Part model, mm, in its own coordinate system. A direction names the side the tool comes from. Round coordinates to 2 decimals unless told otherwise and drop trailing zeros. Write each loop counter-clockwise with the first axis right and the second up, starting at its lowest first coordinate (ties: lowest second). Pieces come first, ordered by that corner, then holes. Notation, with made-up numbers: (45, 31) -> (71, 31) arc R15 cw to (71, 41) -> close; hole circle Ø7 at (-3.5, -32). An arc over 180 degrees is marked (long way). Return JSON: item names as keys, results as strings. Group by question number.
```python
from build123d import *

# Parameters (mm, degrees)
SKETCH1_W                = 25
SKETCH1_H                = 25
BOSS_EXTRUDE1_DEPTH      = 30
SKETCH6_W                = 15
SKETCH6_H                = 15
BOSS_EXTRUDE2_DEPTH      = 8
BOSS_EXTRUDE2_DEPTH_BACK = 12
SKETCH3_R                = 2.5
CUT_EXTRUDE1_DEPTH       = 13.5
CUT_EXTRUDE1_DEPTH_BACK  = 13.5
SKETCH5_R                = 6
CUT_EXTRUDE4_DEPTH       = 11
SKETCH2_R                = 3
CUT_EXTRUDE6_DEPTH       = 31
SKETCH4_R                = 4.25
CUT_EXTRUDE3_DEPTH       = 17.5
FILLET1_R                = 5
FILLET2_R                = 2


with BuildPart() as part:
    # Sketch1 → Boss-Extrude1 (new body)
    with BuildSketch(Plane(origin=(0, 0, 0), x_dir=(1, 0, 0), z_dir=(0, 1, 0))):
        Rectangle(SKETCH1_W, SKETCH1_H)
    extrude(amount=-BOSS_EXTRUDE1_DEPTH)

    # Sketch6 → Boss-Extrude2 (add, two sides)
    with BuildSketch(Plane(origin=(0, 0, 0), x_dir=(1, 0, 0), z_dir=(0, 1, 0))) as boss_extrude2_sk:
        with Locations((20, 5)):
            Rectangle(SKETCH6_W, SKETCH6_H)
        with Locations((-20, 5)):
            Rectangle(SKETCH6_W, SKETCH6_H)
    extrude(amount=BOSS_EXTRUDE2_DEPTH)
    extrude(boss_extrude2_sk.sketch, amount=-BOSS_EXTRUDE2_DEPTH_BACK)

    # Sketch3 → Cut-Extrude1 (cut, two sides)
    with BuildSketch(Plane.XY) as cut_extrude1_sk:
        with Locations((0, -20)):
            Circle(SKETCH3_R)
        with Locations((20, 0)):
            Circle(SKETCH3_R)
        with Locations((-20, 0)):
            Circle(SKETCH3_R)
    extrude(amount=CUT_EXTRUDE1_DEPTH, mode=Mode.SUBTRACT)
    extrude(cut_extrude1_sk.sketch, amount=-CUT_EXTRUDE1_DEPTH_BACK, mode=Mode.SUBTRACT)

    # Sketch5 → Cut-Extrude4 (cut)
    with BuildSketch(Plane.XY.offset(12.5)):
        with Locations((0, -20)):
            Circle(SKETCH5_R)
    extrude(amount=-CUT_EXTRUDE4_DEPTH, mode=Mode.SUBTRACT)

    # Sketch2 → Cut-Extrude6 (cut, through all)
    with BuildSketch(Plane(origin=(0, 0, 0), x_dir=(1, 0, 0), z_dir=(0, 1, 0))):
        with Locations((0, 0.5)):
            Circle(SKETCH2_R)
    extrude(amount=-CUT_EXTRUDE6_DEPTH, mode=Mode.SUBTRACT)

    # Sketch4 → Cut-Extrude3 (cut)
    with BuildSketch(Plane.XZ.offset(30)):
        with Locations((0, -0.5)):
            Circle(SKETCH4_R)
    extrude(amount=-CUT_EXTRUDE3_DEPTH, mode=Mode.SUBTRACT)

    # Fillet1
    fillet1_edges = [part.edges().sort_by_distance(p)[0] for p in [
        (12.5, -12, -5),
        (-12.5, -12, -5),
    ]]
    fillet(fillet1_edges, radius=FILLET1_R)

    # Fillet2
    fillet2_edges = [part.edges().sort_by_distance(p)[0] for p in [
        (12.5, -6, 2.5),
        (-12.5, -6, 2.5),
    ]]
    fillet(fillet2_edges, radius=FILLET2_R)


solid = part.part
```
Item 1: Cut at C-C (z = -6). Write the cut outline in (x, y), then the cut area to 3 significant figures.
Item 2: Flat gauge pins, fed straight in: P1, Ø2, axis at y = -18.5, z = -1, coming from the +X side; P2, Ø6, axis at x = 17.5, y = 3.5, coming from the +Z side; P3, Ø12.5, axis at x = -1.5, z = -6, coming from the +Y side. Where does each tip first touch, or does it go through?
Item 3: Cut at A-A (y = 6.5). Write the cut outline in (x, z).
Item 4: Cut at B-B (x = 0). Write the cut outline in (y, z), then the cut area to 4 significant figures.
Item 5: Wall check: L1, parallel to Y at x = 20, z = -7.5; L2, parallel to X at y = 5, z = 0.5; L3, parallel to Z at x = 23, y = -10. Give the ranges that are in metal, low to high.
Item 6: Which spindle directions (+Z, -Z, +X, -X, +Y, -Y) get a long thin tool onto all of the face, cutting with end or side? Do faces 1 (the face through (22, -12, -5)), 2 (the face through (-12.5, 4, -5)), 3 (the face through (12.5, -18, 3)). Say none if no direction does.
Item 7: Cut at D-D (y = -9). Write the cut outline in (x, z), then the cut area to 3 significant figures.
Item 8: Two-plate mould, pull along Y, no slides. Class faces 4 (the face through (12.5, 4, -5)), 5 (the face through (-3, -30, 3)), 6 (the face through (5, -20, 1.5)): released by +Y, released by -Y, zero draft, split by the parting line, or undercut.
Checks:
{
 "1": {"outline": "(-27.5, -12) -> (-17.5, -12) arc R5 cw to (-12.5, -17) -> (-12.5, -30) -> (12.5, -30) -> (12.5, -17) arc R5 cw to (17.5, -12) -> (27.5, -12) -> (27.5, 8) -> (12.5, 8) -> (12.5, 0) -> (-12.5, 0) -> (-12.5, 8) -> (-27.5, 8) -> close; hole circle Ø5 at (-20, 0); hole circle Ø5 at (0, -20); hole circle Ø5 at (20, 0)", "area": "1,300 mm2"},
 "2": {"P1": "stops at x = 12.5", "P2": "stops at z = 2.5", "P3": "stops at y = 0"},
 "3": {"outline": "(-27.5, -12.5) -> (-12.5, -12.5) -> (-12.5, 2.5) -> (-27.5, 2.5) -> close; (12.5, -12.5) -> (27.5, -12.5) -> (27.5, 2.5) -> (12.5, 2.5) -> close"},
 "4": {"outline": "(-30, -12.5) -> (-22.5, -12.5) -> (-22.5, -4.75) -> (-30, -4.75) -> close; (-30, 3.75) -> (-26, 3.75) -> (-26, 12.5) -> (-30, 12.5) -> close; (-17.5, -12.5) -> (0, -12.5) -> (0, -3.5) -> (-12.5, -3.5) -> (-12.5, -4.75) -> (-17.5, -4.75) -> close; (-14, 3.75) -> (-12.5, 3.75) -> (-12.5, 2.5) -> (0, 2.5) -> (0, 12.5) -> (-14, 12.5) -> close", "area": "382.5 mm2"},
 "5": {"L1": "y = -12 to -2.5, 2.5 to 8", "L2": "x = -27.5 to -12.5, 12.5 to 27.5", "L3": "z = -12.5 to 2.5"},
 "6": {"face 1": "+Z, -Z, +X, -Y", "face 2": "+Z, -Z, +Y", "face 3": "+Z, +X, -Y"},
 "7": {"outline": "(-27.5, -12.5) -> (27.5, -12.5) -> (27.5, 2.5) -> (14.5, 2.5) arc R2 cw to (12.5, 4.5) -> (12.5, 12.5) -> (-12.5, 12.5) -> (-12.5, 4.5) arc R2 cw to (-14.5, 2.5) -> (-27.5, 2.5) -> close; hole circle Ø6 at (0, -0.5)", "area": "1,050 mm2"},
 "8": {"face 4": "zero draft", "face 5": "released by -Y", "face 6": "undercut"}
}
